Check sheet for the modelled part. Datum: model origin and axes. Units: mm. A direction names the side the tool comes from. Round coordinates to 2 decimals unless told otherwise and drop trailing zeros. Order: outer loops, then holes, each group sorted by start corner. A loop starts at its lowest first (then second) coordinate and runs counter-clockwise, first axis right, second up.
from build123d import *

# Parameters (mm, degrees)
SKETCH_1_W               = 600
SKETCH_1_H               = 1200
EXTRUDE_1_DEPTH          = 2000
SKETCH_2_R               = 25
EXTRUDE_2_DEPTH          = 80
MIRROR_2_COPY_1_SKETCH_R = 25
MIRROR_2_COPY_1_DEPTH    = 80


with BuildPart() as part:
    # 草图1 → 凸台-拉伸1 (new body)
    with BuildSketch(Plane(origin=(0, 0, 0), x_dir=(1, 0, 0), z_dir=(0, 1, 0))):
        Rectangle(SKETCH_1_W, SKETCH_1_H)
    extrude(amount=EXTRUDE_1_DEPTH)

    # 草图2 → 凸台-拉伸2 (add)
    with BuildSketch(Plane.XZ):
        with Locations((275, 575)):
            Circle(SKETCH_2_R)
    extrude_2 = extrude(amount=EXTRUDE_2_DEPTH)

    # 镜向1: 凸台-拉伸2 across plane
    add(extrude_2.mirror(Plane(origin=(0, 0, 0), x_dir=(0, 0, 1), z_dir=(1, 0, 0))))

    # 镜向2: 凸台-拉伸2 across plane
    add(extrude_2.mirror(Plane.XY))

    # 镜向2 copy 1 sketch → 镜向2 copy 1 (add)
    with BuildSketch(Plane(origin=(0, 0, 0), x_dir=(-1, 0, 0), z_dir=(0, -1, 0))):
        with Locations((275, 575)):
            Circle(MIRROR_2_COPY_1_SKETCH_R)
    extrude(amount=MIRROR_2_COPY_1_DEPTH)


solid = part.part
1) Sectioned sample at B-B on z = -48.5. Record the cut outline in (x, y).
2) Gauge pin test, flat end, axial feed: pin 1 (5 mm diameter, centred on x = -179, z = -151, fed in from -Y). Record the tip position at first contact, or that the pin passes through.
3) Set-up check for faces 4 (the face through (-275, -80, 575)), 5 (the face through (298.846, -39.44, 582.509)): record each of +Z, -Z, +X, -X, +Y, -Y from which the full face is reachable in a straight line by a thin tool's end or side.
4) Sectioned sample at A-A on x = 60.5. Record the cut outline in (y, z).
5) Draft check along Y on faces 1 (the face through (-4, 2000, -8)), 2 (the face through (-4, 986, -600)), 3 (the face through (-275, -80, -575)). Enter one of: pulls with the +Y half, pulls with the -Y half, needs draft (parallel to the pull), parting line crosses it, or undercut.
6) Scan line: line 1 (Y direction, x = -273, z = 6). Record every from-to range of solid material in increasing order.
Values found:
1. outline: (-300, 0) - (300, 0) - (300, 2000) - (-300, 2000) - close
2. pin 1: stops at y = 0
3. face 4: +Z, -Z, +X, -X, -Y
3. face 5: -Y
4. outline: (0, -600) - (2000, -600) - (2000, 600) - (0, 600) - close
5. face 1: pulls with the +Y half
5. face 2: needs draft
5. face 3: pulls with the -Y half
6. line 1: y = 0 to 2000
